from build123d import *

# Parameters (mm, degrees)
F3_DEPTH      = 17.001
F3_DEPTH_BACK = 25
F5_ANGLE      = -180
F7_DEPTH      = 1.8
F8_DEPTH      = 2.5
F9_R          = 2


with BuildPart() as f1:
    # F0 (on Front) → F1 (revolve)
    with BuildSketch(Plane.XZ):
        with BuildLine():
            Line((-27, 17), (-30, 17))
            Line((-30, 17), (-30, 0))
            Line((-30, 0), (-46.3279513852, 0))
            ThreePointArc((-46.3279513852, 0), (-44.8634852911, -3.5355339059), (-41.3279513852, -5))
            Line((-41.3279513852, -5), (-29, -5))
            ThreePointArc((-29, -5), (-27.5857864376, -4.4142135624), (-27, -3))
            Line((-27, -3), (-27, 17))
        make_face()
    revolve(axis=Axis((0, 0, 7.2955568321), (0, 0, 1)))

    # F2 (on Top) → F3 (cut, two sides)
    with BuildSketch(Plane.XY) as f3_sk:
        Polygon((55.203495074, 0), (0, 0), (55.203495074, -31.8717527412), align=None)
    extrude(amount=F3_DEPTH, mode=Mode.SUBTRACT)
    extrude(f3_sk.sketch, amount=-F3_DEPTH_BACK, mode=Mode.SUBTRACT)


with BuildPart() as f1_1:
    # F5: moved
    add(f1.part.rotate(Axis((0, 0, 17), (0, 0, -1)), F5_ANGLE))

    # F6 (on offset) → F7 (join, symmetric)
    with BuildSketch(Plane.XY.offset(8)):
        with BuildLine():
            ThreePointArc((23.1822198309, -6.2116570825), (22.1731087803, -9.1844023768), (20.7846096908, -12))
            Line((20.7846096908, -12), (24.0563691046, -13.8889511783))
            Line((24.0563691046, -13.8889511783), (26.818160989, -7.1859045795))
            Line((26.818160989, -7.1859045795), (23.1822198309, -6.2116570825))
        make_face()
    extrude(amount=F7_DEPTH, both=True)

    # F6 (on offset) → F8 (cut, symmetric)
    with BuildSketch(Plane.XY.offset(8)):
        Polygon((-34.1305090562, -19.7052585912), (0, 0), (-34.9063649774, 6.3153640367), align=None)
    extrude(amount=F8_DEPTH, both=True, mode=Mode.SUBTRACT)

    # F9
    f9_edges = [f1_1.edges().sort_by_distance(p)[0] for p in [
        (-28.5, 0, 5.5),
        (-28.5, 0, 10.5),
        (-28.5, 0, 17),
        (-24.681724, 14.25, 17),
    ]]
    fillet(f9_edges, radius=F9_R)


solid = f1_1.part
CAD build for the part. Positions are in the model's coordinates, mm. A direction names the side the tool comes from. Give positions to 0.01 mm unless a question says otherwise; leave off trailing zeros. Loops run counter-clockwise (first coordinate to the right, second up) from the corner with the lowest first, then second, coordinate; pieces in that order, holes last. Notation, with made-up numbers: M 43.5,-0.75 L 69.5,-0.75 A20 cw 69.5,4.25 Z; hole C -1.5,41.5 d4. An arc over 180 degrees is marked long. Answer in a Markdown table with one row per item. Add a question column.
Item 1: Band-saw the part on A-A on x = 0. Give the cut face in (y, z), then the cut area to 3 significant figures.
Item 2: Tool access for faces 1 (the face through (-28.44, -0.6, 11.07)), 2 (the face through (-35, 0, -3)), 3 (the face through (-27, -8, 5.5)), 4 (the face through (-24.368, 14.763, 16.43)): list every direction of +Z, -Z, +X, -X, +Y, -Y with a clear straight run to the whole face (end or side of a thin tool).
Item 3: Band-saw the part on D-D on z = 2. Give the cut face in (x, y), then the cut area to 3 significant figures.
Item 4: Band-saw the part on B-B on z = 8.5. Give the cut face in (x, y), then the cut area to 3 significant figures.
Item 5: Probe probe 1 along Y at (x, z) = (0, 4); probe 2 along Z at (x, y) = (15.5, -28); probe 3 along Y at (x, z) = (-2.5, 6.75). List the from-to ranges inside material, lowest first.
Item 6: Mould opens along Y. For faces 5 (the face through (28.64, -8.93, 8.38)), 6 (the face through (25.78, -8.03, 4.92)), 7 (the face through (-28.44, -0.57, 16.4)), 8 (the face through (30, 0, -5)) say: +Y half, -Y half, draft (parallel to the pull), parting line (faces both ways), or undercut.
Item 7: Drop flat-ended pins along their axis: P1, Ø7, axis at x = -40, z = -2.5, coming from the +Y side; P2, Ø4, axis at x = -0.5, z = 12.5, coming from the +Y side; P3, Ø3, axis at x = -28, z = 13, coming from the +Y side. Give the stop position or say it passes through.
Item 8: Band-saw the part on C-C on y = -4. Give the number of separate pieces and of enclosed holes in the cut face, then the cut area to 3 significant figures.
Reply:
| question | item | result |
|---|---|---|
| 1 | outline | M -46.33,0 A5 ccw -41.33,-5 L -29,-5 A2 ccw -27,-3 L -27,17 L -30,17 L -30,0 Z; M 27,-3 A2 ccw 29,-5 L 41.33,-5 A5 ccw 46.33,0 L 30,0 L 30,17 L 27,17 Z |
| 1 | area | 283 mm^2 |
| 2 | face 1 | -X, +Y |
| 2 | face 2 | +Z, -Z, -X |
| 2 | face 3 | -X |
| 2 | face 4 | +Z, -X |
| 3 | outline | M -30,0 A30 ccw long -25.98,15 L -23.38,13.5 A27 cw long -27,0 Z |
| 3 | area | 492 mm^2 |
| 4 | outline | M -25.98,-15 A30 ccw long -25.98,15 L -23.38,13.5 A27 cw 26.08,-6.99 L 23.18,-6.21 A24 cw 20.78,-12 L 23.38,-13.5 A27 cw -23.38,-13.5 Z |
| 4 | area | 468 mm^2 |
| 5 | probe 1 | y = -30 to -27, 27 to 30 |
| 5 | probe 2 | z = -5 to 0 |
| 5 | probe 3 | y = -29.9 to -26.88, 26.88 to 29.9 |
| 6 | face 5 | parting line |
| 6 | face 6 | undercut |
| 6 | face 7 | +Y half |
| 6 | face 8 | draft |
| 7 | P1 | stops at y = 27.98 |
| 7 | P2 | stops at y = 30 |
| 7 | P3 | stops at y = 0 |
| 8 | separate pieces | 3 |
| 8 | enclosed holes | 0 |
| 8 | area | 270 mm^2 |
